from build123d import *

# Parameters (mm, degrees)
BOSS_EXTRUDE1_DEPTH = 340
SKETCH4_W           = 113.333333333
SKETCH4_H           = 10
CUT_EXTRUDE3_DEPTH  = 24.627416998
SKETCH5_W           = 113.333333334
SKETCH5_H           = 10
CUT_EXTRUDE4_DEPTH  = 33.162950904
FILLET2_R           = 10


with BuildPart() as part:
    # Sketch1 → Boss-Extrude1 (new body)
    with BuildSketch(Plane.XY):
        Polygon((48.461940777, 43.461940777), (49.876154339, 44.876154339), (80.461940777, 14.290367902), (80.461940777, -14.290367902), (37.805086528, -56.947222151), (36.390872965, -55.533008589), (78.461940777, -13.461940777), (78.461940777, 13.461940777), align=None)
    extrude(amount=BOSS_EXTRUDE1_DEPTH)

    # Sketch4 → Cut-Extrude3 (cut, through all)
    with BuildSketch(Plane(origin=(45.961940777, 45.961940777, 0), x_dir=(0, 0, 1), z_dir=(-0.707106781, -0.707106781, 0))):
        with Locations((56.666666667, -8.535533906)):
            Rectangle(SKETCH4_W, SKETCH4_H)
        with Locations((283.333333334, -8.535533906)):
            Rectangle(SKETCH4_W, SKETCH4_H)
    extrude(amount=-CUT_EXTRUDE3_DEPTH, mode=Mode.SUBTRACT)

    # Sketch5 → Cut-Extrude4 (cut, through all)
    with BuildSketch(Plane(origin=(45.961940777, -45.961940777, 0), x_dir=(0, 0, 1), z_dir=(-0.707106781, 0.707106781, 0))):
        with Locations((170, -8.535533906)):
            Rectangle(SKETCH5_W, SKETCH5_H)
    extrude(amount=-CUT_EXTRUDE4_DEPTH, mode=Mode.SUBTRACT)

    # Fillet2
    fillet2_edges = [part.edges().sort_by_distance(p)[0] for p in [
        (80.461940777, 14.290367902, 170),
        (80.461940777, -14.290367902, 170),
        (78.461940777, -13.461940777, 170),
        (78.461940777, 13.461940777, 170),
    ]]
    fillet(fillet2_edges, radius=FILLET2_R)


solid = part.part
Source: CAD feature listing. Evaluate the final solid. Frame: model axes, mm. A direction names the side the tool comes from. Give positions to 0.01 mm unless a question says otherwise; leave off trailing zeros. Write each loop counter-clockwise with the first axis right and the second up, starting at its lowest first coordinate (ties: lowest second). Pieces come first, ordered by that corner, then holes. Notation, with made-up numbers: (56, -16) - (101, -16) arc R18 ccw to (101, -11) - close; hole circle Ø10 at (64, -6.5). An arc over 180 degrees is marked (long way). Write item = value, one per line. Start each with the question number.
Q1. Pin query (flat end, axial travel): pin 1 Ø8 at (x, z) = (59.5, 84) entering from -Y; pin 2 Ø4 at (x, y) = (54, 40) entering from +Z; pin 3 Ø1 at (y, z) = (-10, 283) entering from -X. Return the tip coordinate at first contact, or that it passes through.
Q2. Reachability of faces 5 (the flat face through (73, -20, 0)), 6 (the cylindrical face through (77.68, 13.2, 172.38)) from +Z, -Z, +X, -X, +Y, -Y: full face, straight path, thin tool, end or side. Return the list, or none.
Q3. Material intervals for probe 1 along X at (y, z) = (4.5, 120); probe 2 along Y at (x, z) = (64.5, 82); probe 3 along Y at (x, z) = (60, 137), sorted ascending.
Q4. Draft query along Z for faces 1 (the flat face through (41, -53, 226.667)), 2 (the flat face through (73, -20, 340)), 3 (the flat face through (66.58, 28.17, 167.62)), 4 (the flat face through (41, -53, 113.333)). Return one class per face: +Z half, -Z half, draft (parallel to the pull), parting line (faces both ways), or undercut.
Q5. Cut plane D-D, the plane y = -13.5. Return loops of the section in (x, z).
Q6. Cut plane B-B, the plane z = 216. Return loops of the section in (x, y), then the cut area to 3 significant figures.
Q7. Cut plane A-A, the plane x = 62.5. Return loops of the section in (y, z).
Q8. Cut plane C-C, the plane y = 32. Return loops of the section in (x, z), then the cut area to 3 significant figures.
Computed values:
q1.pin_1 = -39.25
q1.pin_2 = 226.67
q1.pin_3 = 78.39
q2.face_5 = -Z, +X, -X, +Y, -Y
q2.face_6 = +Z, -Z, -X
q3.probe_1 = 78.46 to 80.46
q3.probe_2 = -30.25 to -27.42, 27.42 to 30.25
q3.probe_3 = -34.75 to -31.92, 31.92 to 34.75
q4.face_1 = undercut
q4.face_2 = +Z half
q4.face_3 = draft
q4.face_4 = undercut
q5.outline = (77.55, 0) - (79.88, 0) - (79.88, 340) - (77.55, 340) - close
q6.outline = (43.46, -48.46) - (44.88, -49.88) - (77.53, -17.22) arc R10 ccw to (80.46, -10.15) - (80.46, 10.15) arc R10 ccw to (77.53, 17.22) - (49.88, 44.88) - (48.46, 43.46) - (75.53, 16.39) arc R10 cw to (78.46, 9.32) - (78.46, -9.32) arc R10 cw to (75.53, -16.39) - close
q6.area = 241 mm²
q7.outline = (-32.25, 0) - (-29.42, 0) - (-29.42, 340) - (-32.25, 340) - close; (29.42, 0) - (32.25, 0) - (32.25, 340) - (29.42, 340) - close
q8.outline = (59.92, 0) - (62.75, 0) - (62.75, 340) - (59.92, 340) - close
q8.area = 962 mm²
